Verification items for the finished model (mm, model axes). Face numbers are marked on the shaded views. A direction names the side the tool comes from. Coordinates: 2 decimals unless noted, no trailing zeros. Order: outer loops, then holes, each group sorted by start corner. A loop starts at its lowest first (then second) coordinate and runs counter-clockwise, first axis right, second up. Notation, with made-up numbers: (-2, -25.5) - (5, -25.5) arc R16 ccw to (5, -11.5) - close; hole circle Ø10 at (8, -23.5). An arc over 180 degrees is marked (long way). Answer as CSV lines item,"result". Start each with the question number.
1. Material ranges on L1, parallel to X at y = 2.9, z = 20; L2, parallel to Y at x = 4, z = 1.5; L3, parallel to X at y = 0.5, z = 19.5, recorded low to high. Write a range as [from, to].
2. Set-up check for the marked faces 1, 2, 3, 4 and 5: record each of +Z, -Z, +X, -X, +Y, -Y from which the full face is reachable in a straight line by a thin tool's end or side.
3. Go/stop test with flat-tipped pins: pin 1 (5 mm diameter, centred on x = 30, z = 20, fed in from +Y); pin 2 (6.5 mm diameter, centred on x = 0, y = -57, fed in from +Z); pin 3 (6 mm diameter, centred on y = -38, z = -21.5, fed in from -X); pin 4 (5 mm diameter, centred on y = -32.5, z = -21.5, fed in from +X). Record where each tip stops, or that it passes through.
4. Section check C-C (y = -57). Record the cut outline in (x, z), and give its area (3 significant figures).
5. Section check A-A (x = 0). Record the cut outline in (y, z), and give its area (3 significant figures).
6. Section check B-B (z = 20). Record the cut outline in (x, y), and give its area (3 significant figures).
7. Section check D-D (x = 30). Record the cut outline in (y, z).
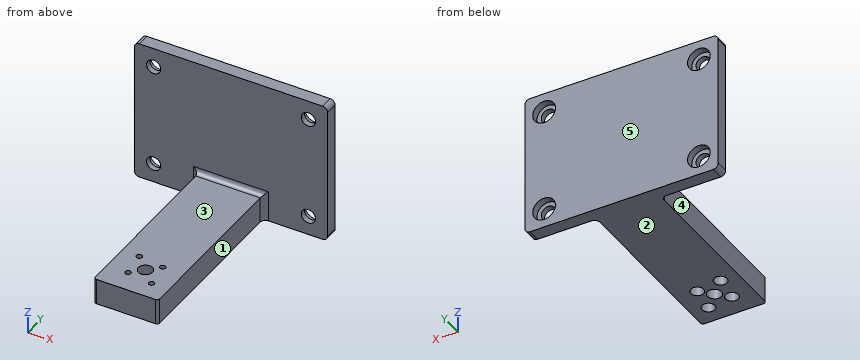
from build123d import *

# Parameters (mm, degrees)
SKETCH1_W           = 75
SKETCH1_H           = 55
BOSS_EXTRUDE1_DEPTH = 5
SKETCH2_R           = 2.75
CUT_EXTRUDE1_DEPTH  = 6
FILLET5_R           = 2
SKETCH6_R           = 4.4
CUT_EXTRUDE3_DEPTH  = 2.8
SKETCH7_W           = 25
SKETCH7_H           = 10
BOSS_EXTRUDE2_DEPTH = 70
SKETCH8_W           = 7
SKETCH8_H           = 30
CUT_EXTRUDE4_DEPTH  = 51
SKETCH11_W          = 25
SKETCH11_H          = 7
BOSS_EXTRUDE3_DEPTH = 30
FILLET6_R           = 2
FILLET7_R           = 1
SKETCH17_R          = 2.75
SKETCH17_R_2        = 1.1
CUT_EXTRUDE5_DEPTH  = 56
SKETCH18_R          = 2.5
CUT_EXTRUDE6_DEPTH  = 7


with BuildPart() as part:
    # Sketch1 → Boss-Extrude1 (new body)
    with BuildSketch(Plane(origin=(0, 0, 0), x_dir=(1, 0, 0), z_dir=(0, 1, 0))):
        Rectangle(SKETCH1_W, SKETCH1_H)
    extrude(amount=BOSS_EXTRUDE1_DEPTH)

    # Sketch2 → Cut-Extrude1 (cut, through all)
    with BuildSketch(Plane(origin=(0, 5, 0), x_dir=(1, 0, 0), z_dir=(0, 1, 0))):
        with Locations((-30, 20)):
            Circle(SKETCH2_R)
        with Locations((-30, -20)):
            Circle(SKETCH2_R)
    cut_extrude1 = extrude(amount=-CUT_EXTRUDE1_DEPTH, mode=Mode.SUBTRACT)

    # Mirror1: Cut-Extrude1 across plane
    add(cut_extrude1.mirror(Plane(origin=(0, 0, 0), x_dir=(0, 0, 1), z_dir=(1, 0, 0))), mode=Mode.SUBTRACT)

    # Fillet5
    fillet5_edges = [part.edges().sort_by_distance(p)[0] for p in [
        (37.5, 2.5, 27.5),
        (-37.5, 2.5, 27.5),
        (-37.5, 2.5, -27.5),
        (37.5, 2.5, -27.5),
    ]]
    fillet(fillet5_edges, radius=FILLET5_R)

    # Sketch6 → Cut-Extrude3 (cut)
    with BuildSketch(Plane(origin=(0, 5, 0), x_dir=(1, 0, 0), z_dir=(0, 1, 0))):
        with Locations((-30, 20)):
            Circle(SKETCH6_R)
        with Locations((-30, -20)):
            Circle(SKETCH6_R)
        with Locations((30, 20)):
            Circle(SKETCH6_R)
        with Locations((30, -20)):
            Circle(SKETCH6_R)
    extrude(amount=-CUT_EXTRUDE3_DEPTH, mode=Mode.SUBTRACT)

    # Sketch7 → Boss-Extrude2 (add)
    with BuildSketch(Plane.XZ):
        with Locations((0, -22.5)):
            Rectangle(SKETCH7_W, SKETCH7_H)
    extrude(amount=BOSS_EXTRUDE2_DEPTH)

    # Sketch8 → Cut-Extrude4 (cut, through all)
    with BuildSketch(Plane.ZY.offset(12.5)):
        with Locations((-21, -55)):
            Rectangle(SKETCH8_W, SKETCH8_H)
    extrude(amount=-CUT_EXTRUDE4_DEPTH, mode=Mode.SUBTRACT)

    # Sketch11 → Boss-Extrude3 (add)
    with BuildSketch(Plane.XZ.offset(40)):
        with Locations((0, -21)):
            Rectangle(SKETCH11_W, SKETCH11_H)
    extrude(amount=BOSS_EXTRUDE3_DEPTH)

    # Fillet6
    fillet6_edges = [part.edges().sort_by_distance(p)[0] for p in [
        (-12.5, 0, -22.5),
        (12.5, 0, -22.5),
        (0, 0, -17.5),
    ]]
    fillet(fillet6_edges, radius=FILLET6_R)

    # Fillet7
    fillet7_edges = [part.edges().sort_by_distance(p)[0] for p in [
        (12.5, -70, -22.5),
        (-12.5, -70, -22.5),
    ]]
    fillet(fillet7_edges, radius=FILLET7_R)

    # Sketch17 → Cut-Extrude5 (cut, through all)
    with BuildSketch(Plane(origin=(0, 0, -27.5), x_dir=(-1, 0, 0), z_dir=(0, 0, -1))):
        with Locations((0, -57)):
            Circle(SKETCH17_R)
        with Locations((5.656854249, -51.343145751)):
            Circle(SKETCH17_R_2)
        with Locations((-5.656854249, -62.656854249)):
            Circle(SKETCH17_R_2)
        with Locations((-4.242640687, -52.757359313)):
            Circle(SKETCH17_R_2)
        with Locations((4.242640687, -61.242640687)):
            Circle(SKETCH17_R_2)
    extrude(amount=-CUT_EXTRUDE5_DEPTH, mode=Mode.SUBTRACT)

    # Sketch18 → Cut-Extrude6 (cut)
    with BuildSketch(Plane(origin=(0, 0, -27.5), x_dir=(-1, 0, 0), z_dir=(0, 0, -1))):
        with Locations((-4.242640687, -52.757359313)):
            Circle(SKETCH18_R)
        with Locations((-5.656854249, -62.656854249)):
            Circle(SKETCH18_R)
        with Locations((5.656854249, -51.343145751)):
            Circle(SKETCH18_R)
        with Locations((4.242640687, -61.242640687)):
            Circle(SKETCH18_R)
    extrude(amount=-CUT_EXTRUDE6_DEPTH, mode=Mode.SUBTRACT)


solid = part.part
Evaluation:
1,L1,"x = [-37.5, -34.4], [-25.6, 25.6], [34.4, 37.5]"
1,L2,"y = [0, 5]"
1,L3,"x = [-37.5, -32.7], [-27.3, 27.3], [32.7, 37.5]"
2,face 1,"+Z, -Z, +X, -Y"
2,face 2,"-Z, +X, -X, +Y, -Y"
2,face 3,"+Z, +X, -X, -Y"
2,face 4,"+Z, -Z, -X, -Y"
2,face 5,"+Z, -Z, +X, -X, +Y"
3,pin 1,"passes through"
3,pin 2,"stops at z = -17.5"
3,pin 3,"stops at x = -12.5"
3,pin 4,"stops at x = 12.5"
4,outline,"(-12.5, -27.5) - (-2.75, -27.5) - (-2.75, -17.5) - (-12.5, -17.5) - close; (2.75, -27.5) - (12.5, -27.5) - (12.5, -17.5) - (2.75, -17.5) - close"
4,area,"195 mm²"
5,outline,"(-70, -27.5) - (-59.75, -27.5) - (-59.75, -17.5) - (-70, -17.5) - close; (-54.25, -27.5) - (5, -27.5) - (5, 27.5) - (0, 27.5) - (0, -15.5) arc R2 cw to (-2, -17.5) - (-54.25, -17.5) - close"
5,area,"921 mm²"
6,outline,"(-37.5, 0) - (-32.75, 0) - (-32.75, 2.2) - (-34.4, 2.2) - (-34.4, 5) - (-37.5, 5) - close; (-27.25, 0) - (27.25, 0) - (27.25, 2.2) - (25.6, 2.2) - (25.6, 5) - (-25.6, 5) - (-25.6, 2.2) - (-27.25, 2.2) - close; (32.75, 0) - (37.5, 0) - (37.5, 5) - (34.4, 5) - (34.4, 2.2) - (32.75, 2.2) - close"
6,area,"302 mm²"
7,outline,"(0, -27.5) - (5, -27.5) - (5, -24.4) - (2.2, -24.4) - (2.2, -22.75) - (0, -22.75) - close; (0, -17.25) - (2.2, -17.25) - (2.2, -15.6) - (5, -15.6) - (5, 15.6) - (2.2, 15.6) - (2.2, 17.25) - (0, 17.25) - close; (0, 22.75) - (2.2, 22.75) - (2.2, 24.4) - (5, 24.4) - (5, 27.5) - (0, 27.5) - close"
